```python
from build123d import *

# Parameters (mm, degrees)
BOSS_EXTRUDE1_DEPTH = 298.45
CUT_EXTRUDE1_DEPTH  = 711.2
SKETCH3_R           = 1.5
CUT_EXTRUDE2_DEPTH  = 711.2


with BuildPart() as part:
    # Sketch1 → Boss-Extrude1 (new body)
    with BuildSketch(Plane.XY):
        Polygon((0, 25.4), (0, 0), (25.4, 0), (25.4, 3.175), (3.175, 3.175), (3.175, 25.4), align=None)
    extrude(amount=BOSS_EXTRUDE1_DEPTH)

    # Sketch2 → Cut-Extrude1 (cut)
    with BuildSketch(Plane.ZY):
        Polygon((0, 8.542079309), (0, 0), (25.4, 25.4), (0, 25.4), align=None)
        Polygon((298.45, 25.4), (273.05, 25.4), (298.45, 0), align=None)
    extrude(amount=-CUT_EXTRUDE1_DEPTH, mode=Mode.SUBTRACT)

    # Sketch3 → Cut-Extrude2 (cut)
    with BuildSketch(Plane.XZ):
        with Locations((15.875, 285.75)):
            Circle(SKETCH3_R)
        with Locations((15.875, 12.7)):
            Circle(SKETCH3_R)
    extrude(amount=-CUT_EXTRUDE2_DEPTH, mode=Mode.SUBTRACT)


solid = part.part
```
Source: CAD feature listing. Evaluate the final solid. Frame: model axes, mm. A direction names the side the tool comes from. Round coordinates to 2 decimals unless told otherwise and drop trailing zeros. Write each loop counter-clockwise with the first axis right and the second up, starting at its lowest first coordinate (ties: lowest second). Pieces come first, ordered by that corner, then holes. Notation, with made-up numbers: M 15.25,88.25 L 73.25,88.25 A16 cw 73.25,109.25 Z; hole C 59.25,10 d3. An arc over 180 degrees is marked long. Use CSV: the item, a comma, the result in double quotes. Start each with the question number.
Q1. Cut plane B-B on y = 22. Output: boundary loops of the cut face in (x, z) (3 decimals), plus the area to 3 significant figures.
Q2. Line query: line 1 (X direction, y = 1.8, z = 285.75) (3 decimals); line 2 (Z direction, x = 17, y = 3); line 3 (X direction, y = 16.25, z = 182) (3 decimals). Output: solid intervals per line, ascending. Write a range as from..to.
Q3. Access query for faces 1 (the face through (2, 7, 7)), 2 (the face through (14, 3.175, 147)). Directions: +Z, -Z, +X, -X, +Y, -Y. A direction counts if a zero-diameter tool reaches every point of the face in a straight line with its end or side. Return the directions, or none.
Q4. Cut plane A-A on z = 152. Output: boundary loops of the cut face in (x, y) (3 decimals), plus the area to 3 significant figures.
Q5. Cut plane C-C on y = 8.75. Output: boundary loops of the cut face in (x, z) (3 decimals).
Q6. First-contact query: P1, Ø4, axis at x = 3, y = 4, coming from the +Z side; P2, Ø3, axis at x = 22.5, z = 181, coming from the -Y side; P3, Ø3, axis at y = 7.5, z = 205.5, coming from the +X side (3 decimals); P4, Ø3, axis at x = 9, z = 111, coming from the +Y side (3 decimals). Flat tips, straight axial feed; report the tip coordinate or a pass-through.
Results found:
1,outline,"M 0,22 L 3.175,22 L 3.175,276.45 L 0,276.45 Z"
1,area,"808 mm^2"
2,line 1,"0..14.375, 17.375..25.4"
2,line 2,"3..11.71, 13.69..284.76, 286.74..295.45"
2,line 3,"0..3.175"
3,face 1,"-Z, +X, -X, +Y"
3,face 2,"+Z, -Z, +X, +Y"
4,outline,"M 0,0 L 25.4,0 L 25.4,3.175 L 3.175,3.175 L 3.175,25.4 L 0,25.4 Z"
4,area,"151 mm^2"
5,outline,"M 0,8.75 L 3.175,8.75 L 3.175,289.7 L 0,289.7 Z"
6,P1,"z = 296.45"
6,P2,"y = 0"
6,P3,"x = 3.175"
6,P4,"y = 3.175"
